Build history of the part. All positions in model axes, mm. A direction names the side the tool comes from. Give positions to 0.01 mm unless a question says otherwise; leave off trailing zeros. Loops run counter-clockwise (first coordinate to the right, second up) from the corner with the lowest first, then second, coordinate; pieces in that order, holes last. Notation, with made-up numbers: (7.25, -5.5) - (42.25, -5.5) arc R26 ccw to (42.25, 21.5) - close; hole circle Ø11 at (65.25, 57). An arc over 180 degrees is marked (long way). Return JSON: item names as keys, results as strings. Group by question number.
1) Mould opens along X. For faces 1 (the face through (-77, 34.5, -2)), 2 (the face through (-82, -31, -2)), 3 (the face through (80, -31, -2)) say: released by +X, released by -X, zero draft, split by the parting line, or undercut.
2) Slice it at B-B (x = 57.5). List the corners of the cut face in (y, z).
3) Slice it at C-C (y = 11.5). List the corners of the cut face in (x, z).
4) Drill centre lines: probe 1 along Y at (x, z) = (78.5, -2.95); probe 2 along X at (y, z) = (-3, -3.35); probe 3 along Y at (x, z) = (-44.5, -2.1). Where is each one in solid material? Low to high. Write a range as from..to.
5) 3-axis set-ups, long thin cutter, end or side, ignore diameter. For faces 4 (the face through (1, -32.5, -2)), 5 (the face through (1, 32.5, -2)), 6 (the face through (75, 0, -2)): which of +Z, -Z, +X, -X, +Y, -Y reach the whole face in a straight line?
6) Slice it at A-A (y = -31). List the corners of the cut face in (x, z).
7) Drop flat-ended pins along their axis: pin 1 (0.6 mm diameter, centred on y = 33.5, z = -2, fed in from +X); pin 2 (2 mm diameter, centred on y = -4.5, z = -3, fed in from +X); pin 3 (1.8 mm diameter, centred on x = 78.5, y = -31, fed in from +Z); pin 4 (0.6 mm diameter, centred on y = -33.5, z = -2, fed in from -X). Give the stop position or say it passes through.
Autodesk Inventor part; units mm, degrees
ref_plane "YZ Plane" through (0, 0, 0) normal (1, 0, 0) x (0, 1, 0)
ref_plane "XZ Plane" through (0, 0, 0) normal (0, 1, 0) x (-1, 0, 0)
ref_plane "XY Plane" through (0, 0, 0) normal (0, 0, 1) x (1, 0, 0)
sketch "Sketch1" plane through (0, 0, 0) normal (0, 0, 1) x (1, 0, 0)
  line L0 (0, 15198.2615) -> (0, -15198.2615) construction
  line L1 (-114.9467, 0) -> (114.9467, 0) construction
  line L2 (0, -32.5) -> (-75, -32.5)
  line L3 (-75, -32.5) -> (-75, -34.5)
  circle A0 centre (-78.5, -31) radius 1.5
  line L4 (-75, -34.5) -> (-78.5, -34.5)
  arc A1 (-78.7128, -27.5065) -> (-78.5, -34.5) centre (-78.5, -31) ccw
  line L5 (-75, -22.5739) -> (-75, 0)
  line L6 (-78.7128, -27.5065) -> (-75, -27.2803) construction
  line L7 (-75, -27.2803) -> (-75, -22.5739) construction
  spline S0 degree 2 poles (-78.7128, -27.5065) (-75, -27.2803) (-75, -22.5739) knots 1 1 1 2 2 2
  line L8 (0, -32.5) -> (75, -32.5)
  line L9 (75, -32.5) -> (75, -34.5)
  circle A2 centre (78.5, -31) radius 1.5
  line L10 (75, -34.5) -> (78.5, -34.5)
  arc A3 (78.5, -34.5) -> (78.7128, -27.5065) centre (78.5, -31) ccw
  line L11 (75, -22.5739) -> (75, 0)
  line L12 (78.7128, -27.5065) -> (75, -27.2803) construction
  line L13 (75, -27.2803) -> (75, -22.5739) construction
  spline S1 degree 2 poles (78.7128, -27.5065) (75, -27.2803) (75, -22.5739) knots 1 1 1 2 2 2
  line L14 (0, -15198.2615) -> (0, 15198.2615) construction
  line L15 (0, 32.5) -> (-75, 32.5)
  line L16 (-75, 32.5) -> (-75, 34.5)
  circle A4 centre (-78.5, 31) radius 1.5
  line L17 (-75, 34.5) -> (-78.5, 34.5)
  arc A5 (-78.5, 34.5) -> (-78.7128, 27.5065) centre (-78.5, 31) ccw
  line L18 (-75, 22.5739) -> (-75, 0)
  line L19 (-78.7128, 27.5065) -> (-75, 27.2803) construction
  line L20 (-75, 27.2803) -> (-75, 22.5739) construction
  spline S2 degree 2 poles (-78.7128, 27.5065) (-75, 27.2803) (-75, 22.5739) knots 1 1 1 2 2 2
  line L21 (0, 32.5) -> (75, 32.5)
  line L22 (75, 32.5) -> (75, 34.5)
  circle A6 centre (78.5, 31) radius 1.5
  line L23 (75, 34.5) -> (78.5, 34.5)
  arc A7 (78.7128, 27.5065) -> (78.5, 34.5) centre (78.5, 31) ccw
  line L24 (75, 22.5739) -> (75, 0)
  line L25 (78.7128, 27.5065) -> (75, 27.2803) construction
  spline S3 degree 2 poles (78.7128, 27.5065) (75, 27.2803) (75, 22.5739) knots 1 1 1 2 2 2
  line L26 (75, 27.2803) -> (75, 22.5739) construction
  point P0 (0, 0)
  dimension "d0" = 2
  dimension "d1" = 3
  dimension "d3" = 75
  dimension "d4" = 32.5
  dimension "d5" = 3.5
  dimension "d6" = 3.5
extrude "Extrusion1" add sketch "Sketch1" against normal blind 5
equation "\"d0\" = Cover_Thickness"
equation "\"d3\" = 0.5 * Heatsink_Length"
equation "\"d4\" = 0.5 * Heatsink_Width"
equation "\"d6\" = d5"
equation "\"d7\" = Heatsink_Thickness"
equation "\"Heatsink_Thickness\" = 5"
equation "\"Cover_Thickness\" = 2"
equation "\"Heatsink_Width\" = 65"
equation "\"PowerPCB_Minus_Height\" = 1.2"
equation "\"PowerPCB_Width\" = 63"
equation "\"Interface_Thickness\" = 7"
equation "\"PowerPCB_Thickness\" = 3"
equation "\"PowerPCB_Plus_Height\" = 8"
equation "\"LogicPCB_Width\" = 55"
equation "\"LogicPCB_Thickness\" = 2"
equation "\"LogicPCB_Plus_Height\" = 8"
equation "\"HostPCB_Plus_Height\" = 8"
equation "\"HostPCB_Thickness\" = 1.2"
properties part number "Heatsink" material "Aluminum 6061"
Results:
{
 "1": {"face 1": "zero draft", "face 2": "released by -X", "face 3": "undercut"},
 "2": {"outline": "(-32.5, -5) - (32.5, -5) - (32.5, 0) - (-32.5, 0) - close"},
 "3": {"outline": "(-75, -5) - (75, -5) - (75, 0) - (-75, 0) - close"},
 "4": {"probe 1": "-34.5..-32.5, -29.5..-27.49, 27.49..29.5, 32.5..34.5", "probe 2": "-75..75", "probe 3": "-32.5..32.5"},
 "5": {"face 4": "+Z, -Z, -Y", "face 5": "+Z, -Z, +Y", "face 6": "+Z, -Z, +X"},
 "6": {"outline": "(-82, -5) - (-80, -5) - (-80, 0) - (-82, 0) - close; (-77, -5) - (77, -5) - (77, 0) - (-77, 0) - close; (80, -5) - (82, -5) - (82, 0) - (80, 0) - close"},
 "7": {"pin 1": "x = 81.22", "pin 2": "x = 75", "pin 3": "through", "pin 4": "x = -81.22"}
}
